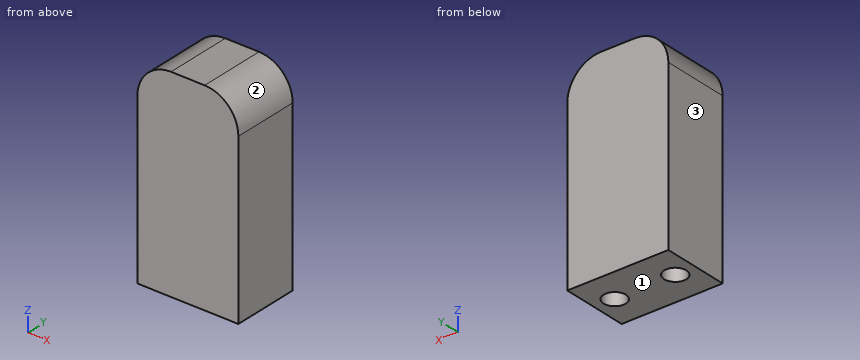
```python
from build123d import *

# Parameters (mm, degrees)
F0_W     = 15
F0_H     = 30
F1_DEPTH = 10
F3_D     = 3.3
F3_DEPTH = 10
F3_TIP   = 0.9914200214
F4_R     = 5


with BuildPart() as f1:
    # F0 (on Front) → F1 (new body)
    with BuildSketch(Plane.XZ):
        with Locations((0, 15)):
            Rectangle(F0_W, F0_H)
    extrude(amount=F1_DEPTH)

    # F3
    with Locations(Plane(origin=(0, 0, 0), x_dir=(1, 0, 0), z_dir=(0, 0, -1))):
        with Locations((-4.5, 5), (4.5, 5)):
            Hole(F3_D / 2, depth=F3_DEPTH)
            with Locations((0, 0, -(F3_DEPTH + F3_TIP / 2))):  # 118° drill point
                Cone(0, F3_D / 2, F3_TIP, mode=Mode.SUBTRACT)

    # F4
    f4_edges = [f1.edges().sort_by_distance(p)[0] for p in [
        (-7.5, -5, 30),
        (7.5, -5, 30),
    ]]
    fillet(f4_edges, radius=F4_R)


solid = f1.part
```
Here's how the part is built. I have some questions about the finished solid (model axes, mm). Face numbers are marked on the shaded views. Coordinates: 2 decimals unless noted, no trailing zeros. Loops run counter-clockwise (first coordinate to the right, second up) from the corner with the lowest first, then second, coordinate; pieces in that order, holes last. Notation, with made-up numbers: (75, 74.25) - (94, 74.25) arc R20 cw to (94, 109.25) - close; hole circle Ø11 at (70.25, -38). An arc over 180 degrees is marked (long way). Answer as CSV lines item,"result".
Q1. If we section it at C-C, the plane x = -6.5: Write out the boundary of the cut face in (y, z).
Response:
outline,"(-10, 0) - (0, 0) - (0, 28) - (-10, 28) - close"
Q2. If I drill on L1, parallel to X at y = -5, z = 7; L2, parallel to Y at x = -4.5, z = 5; L3, parallel to Y at x = -3.75, z = 8.75, over which ranges is the centre line in solid material (lowest first)? Write a range as [from, to].
Response:
L1,"[-7.5, -6.15], [-2.85, 2.85], [6.15, 7.5]"
L2,"[-10, -6.65], [-3.35, 0]"
L3,"[-10, -6.47], [-3.53, 0]"
Q3. We'd pull the mould along Z, two halves only. Please class the marked faces 1, 2 and 3: pulls with the +Z half, pulls with the -Z half, needs draft (parallel to the pull), parting line crosses it, or undercut.
Response:
face 1,"pulls with the -Z half"
face 2,"pulls with the +Z half"
face 3,"needs draft"
Q4. If we section it at B-B, the plane y = -0.5: Write out the boundary of the cut face in (x, z), and give its area (3 significant figures).
Response:
outline,"(-7.5, 0) - (7.5, 0) - (7.5, 25) arc R5 ccw to (2.5, 30) - (-2.5, 30) arc R5 ccw to (-7.5, 25) - close"
area,"439 mm2"
Q5. If we section it at A-A, the plane z = 2.5: Write out the boundary of the cut face in (x, y).
Response:
outline,"(-7.5, -10) - (7.5, -10) - (7.5, 0) - (-7.5, 0) - close; hole circle Ø3.3 at (-4.5, -5); hole circle Ø3.3 at (4.5, -5)"
Q6. For pin 1 (2.5 mm diameter, centred on x = 4.5, y = -5, fed in from -Z); pin 2 (3 mm diameter, centred on x = -4.5, y = -5, fed in from -Z); pin 3 (1 mm diameter, centred on x = 3.5, y = -2, fed in from +Z), each with a flat end and sliding along its axis, tell me the tip position at first contact or that it passes through.
Response:
pin 1,"z = 10.24"
pin 2,"z = 10.09"
pin 3,"z = 29.97"
